from build123d import *

# Parameters (mm, degrees)
F1_DEPTH = 57.658
F2_W     = 8.732148
F2_H     = 15.885746
F3_DEPTH = 25.4
F4_W     = 14.180422
F4_H     = 9.618062
F5_DEPTH = 25.4
F6_W     = 57.658
F6_H     = 24.840316
F6_W_2   = 14.180422
F6_H_2   = 9.618062
F6_W_3   = 13.320997
F6_H_3   = 8.912906
F7_DEPTH = 25.4
F8_W     = 16.328969
F8_H     = 7.385209
F9_DEPTH = 25.4


with BuildPart() as f1:
    # F0 (on Front) → F1 (new body)
    with BuildSketch(Plane.XZ):
        Polygon((-18.141802, 0), (-18.141802, -24.840316), (18.886082, -24.840316), (18.886082, 0), (0, 21.304989), align=None)
    extrude(amount=F1_DEPTH)

    # F2 (on face) → F3 (cut)
    with BuildSketch(Plane.XZ.offset(57.658)):
        with Locations((-4.366074, -16.897443)):
            Rectangle(F2_W, F2_H)
    extrude(amount=-F3_DEPTH, mode=Mode.SUBTRACT)

    # F4 (on face) → F5 (cut)
    with BuildSketch(Plane.YZ.offset(18.886082)):
        with Locations((-39.082445, -11.540385)):
            Rectangle(F4_W, F4_H)
    extrude(amount=-F5_DEPTH, mode=Mode.SUBTRACT)

    # F6 (on face) → F7 (join)
    with BuildSketch(Plane.YZ.offset(18.886082)):
        with Locations((-28.829, -12.420158)):
            Rectangle(F6_W, F6_H)
        with Locations((-39.082445, -11.540385)):
            Rectangle(F6_W_2, F6_H_2, mode=Mode.SUBTRACT)
        with Locations((-13.299853, -11.187807)):
            Rectangle(F6_W_3, F6_H_3, mode=Mode.SUBTRACT)
    extrude(amount=F7_DEPTH)

    # F8 (on face) → F9 (cut)
    with BuildSketch(Plane.XZ.offset(57.658)):
        with Locations((20.488108, -15.033167)):
            Rectangle(F8_W, F8_H)
    extrude(amount=-F9_DEPTH, mode=Mode.SUBTRACT)


solid = f1.part
Geometry check sheet. Reference: the model listing, model coordinates, mm. A direction names the side the tool comes from. Coordinates: 2 decimals unless noted, no trailing zeros. Loops run counter-clockwise (first coordinate to the right, second up) from the corner with the lowest first, then second, coordinate; pieces in that order, holes last. Notation, with made-up numbers: (89.5, 66) - (124.5, 66) arc R14 cw to (124.5, 81) - close; hole circle Ø10 at (-7.5, 51.25). An arc over 180 degrees is marked (long way). Use one line per item in the form item = value. Start each with the question number.
Item 1: Mould release check, pull along Y, two halves, no side actions. Record for faces 1 (the face through (9.58, -28.43, 10.5)), 2 (the face through (30, -39, -16.349)), 3 (the face through (20, -32.258, -18)), 4 (the face through (13, 0, -7)): +Y half, -Y half, draft (parallel to the pull), parting line (faces both ways), or undercut.
Item 2: Section check A-A, the plane y = -40. Enter the section's corners in (x, z), and give its area (3 significant figures).
Item 3: Gauge pin test, flat ends, axial feed: pin 1 (18 mm diameter, centred on x = 16.5, y = -39, fed in from +Z); pin 2 (5 mm diameter, centred on y = -40, z = -13, fed in from +X); pin 3 (7 mm diameter, centred on x = -5, y = -40.5, fed in from -Z); pin 4 (9.5 mm diameter, centred on x = -2.5, z = -20, fed in from -Y). Record the tip position at first contact, or that the pin passes through.
Item 4: Section check D-D, the plane x = 25.5. Enter the section's corners in (y, z), and give its area (3 significant figures).
Item 5: Section check B-B, the plane x = 33.5. Enter the section's corners in (y, z), and give its area (3 significant figures).
Item 6: Thickness scan on probe 1 along Z at (x, y) = (23.5, -40.5); probe 2 along Y at (x, z) = (38.5, -9.5); probe 3 along Z at (x, y) = (20, -9). Record the ranges inside material, lowest first.
Item 7: Section check C-C, the plane y = -48.5. Enter the section's corners in (x, z), and give its area (3 significant figures).
Item 8: Tool access check on faces 5 (the face through (31, -6.639, -11)), 6 (the face through (-5, -32.258, -19)), 7 (the face through (13, -29, -24.84)), 8 (the face through (-8.944, -28.425, 10.802)), 9 (the face through (12.324, -48, -16)). Record the directions out of +Z, -Z, +X, -X, +Y, -Y that give a thin tool (end or side, any length) a straight path to the whole face; none if there is none.
Computed:
q1.face_1 = draft
q1.face_2 = undercut
q1.face_3 = -Y half
q1.face_4 = +Y half
q2.outline = (-18.14, -24.84) - (-8.73, -24.84) - (-8.73, -8.95) - (-6.51, -8.95) - (-6.51, -6.73) - (44.29, -6.73) - (44.29, 0) - (18.89, 0) - (0, 21.3) - (-18.14, 0) - close; (0, -24.84) - (44.29, -24.84) - (44.29, -16.35) - (28.65, -16.35) - (28.65, -18.73) - (12.32, -18.73) - (12.32, -16.35) - (0, -16.35) - close
q2.area = 1,330 mm2
q3.pin_1 = 12.84
q3.pin_2 = -8.73
q3.pin_3 = -8.95
q3.pin_4 = -57.66
q4.outline = (-57.66, -24.84) - (0, -24.84) - (0, 0) - (-57.66, 0) - (-57.66, -11.34) - (-46.17, -11.34) - (-46.17, -6.73) - (-31.99, -6.73) - (-31.99, -16.35) - (-32.26, -16.35) - (-32.26, -18.73) - (-57.66, -18.73) - close; hole (-19.96, -15.64) - (-6.64, -15.64) - (-6.64, -6.73) - (-19.96, -6.73) - close
q4.area = 1,060 mm2
q5.outline = (-57.66, -24.84) - (0, -24.84) - (0, 0) - (-57.66, 0) - close; hole (-46.17, -16.35) - (-31.99, -16.35) - (-31.99, -6.73) - (-46.17, -6.73) - close; hole (-19.96, -15.64) - (-6.64, -15.64) - (-6.64, -6.73) - (-19.96, -6.73) - close
q5.area = 1,180 mm2
q6.probe_1 = -24.84 to -18.73, -6.73 to 0
q6.probe_2 = -57.66 to -46.17, -31.99 to -19.96, -6.64 to 0
q6.probe_3 = -24.84 to -15.64, -6.73 to 0
q7.outline = (-18.14, -24.84) - (-8.73, -24.84) - (-8.73, -8.95) - (0, -8.95) - (0, -24.84) - (44.29, -24.84) - (44.29, 0) - (18.89, 0) - (0, 21.3) - (-18.14, 0) - close; hole (12.32, -18.73) - (28.65, -18.73) - (28.65, -11.34) - (12.32, -11.34) - close
q7.area = 1,690 mm2
q8.face_5 = +X
q8.face_6 = -Z, -Y
q8.face_7 = -Z, +X, -X, +Y, -Y
q8.face_8 = +Z, -X, +Y, -Y
q8.face_9 = -Y
